Geometry: see drawing. Coordinates: mm, zero at the bounding-box minimum. A direction names the side the tool comes from. Give positions to 0.01 mm unless a question says otherwise; leave off trailing zeros. Write each loop counter-clockwise with the first axis right and the second up, starting at its lowest first coordinate (ties: lowest second). Pieces come first, ordered by that corner, then holes.
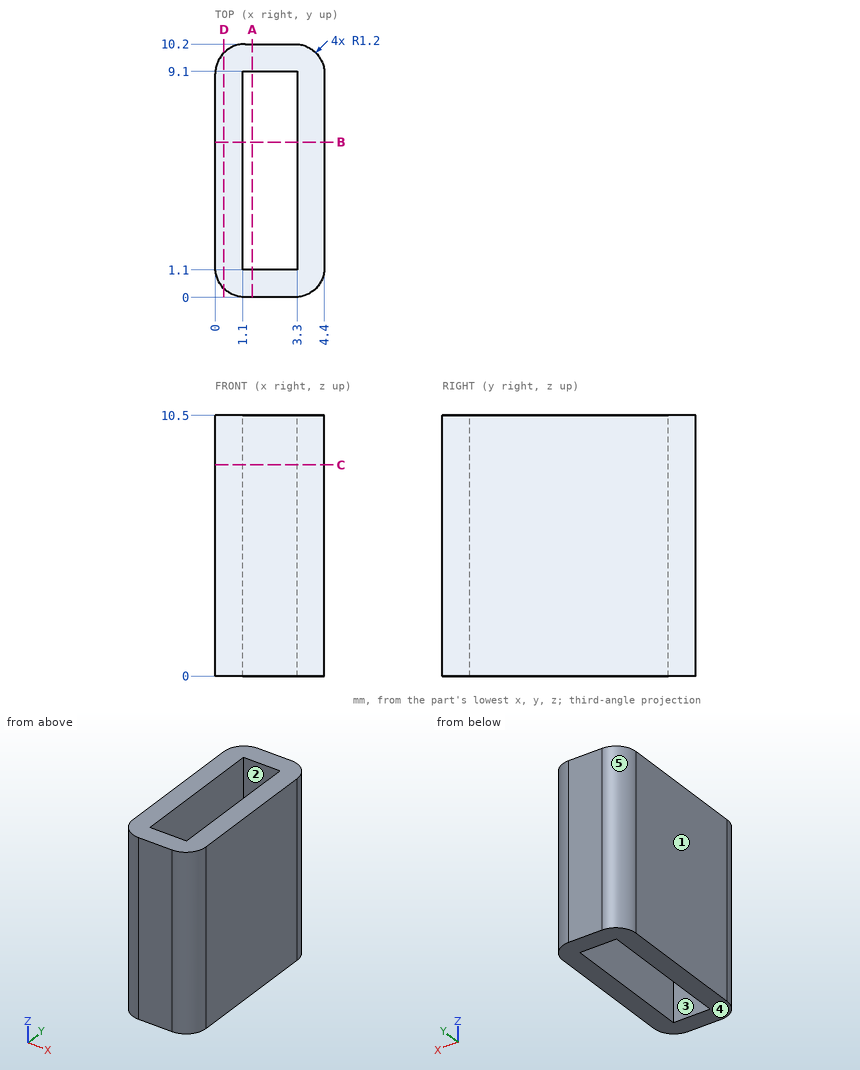
1. Section query A-A (x = 1.5). Return loops of the section in (y, z), plus the area to 3 significant figures.
2. Pull-direction query (X, two-part tool) for the marked faces 3, 4 and 5; classes: pulls with the +X half, pulls with the -X half, needs draft (parallel to the pull), parting line crosses it, or undercut.
3. Section query B-B (y = 6.25). Return loops of the section in (x, z).
4. Section query C-C (z = 8.5). Return loops of the section in (x, y), plus the area to 3 significant figures.
5. Line query: probe 1 along Y at (x, z) = (1.4, 2.75); probe 2 along X at (y, z) = (5.75, 3.5); probe 3 along Y at (x, z) = (0.5, 1.5). Output: solid intervals per line, ascending.
6. Access query for the marked faces 1 and 2. Directions: +Z, -Z, +X, -X, +Y, -Y. A direction counts if a zero-diameter tool reaches every point of the face in a straight line with its end or side. Return the directions, or none.
7. Section query D-D (x = 0.35). Return loops of the section in (y, z), plus the area to 3 significant figures.
8. Pin query (flat end, axial travel): P1, Ø4, axis at y = 6.5, z = 6.5, coming from the -X side. Return the tip coordinate at first contact, or that it passes through.
The answers:
1. outline: (0, 0) - (1.1, 0) - (1.1, 10.5) - (0, 10.5) - close; (9.1, 0) - (10.2, 0) - (10.2, 10.5) - (9.1, 10.5) - close
1. area: 23.1 mm2
2. face 3: undercut
2. face 4: needs draft
2. face 5: pulls with the -X half
3. outline: (0, 0) - (1.1, 0) - (1.1, 10.5) - (0, 10.5) - close; (3.3, 0) - (4.4, 0) - (4.4, 10.5) - (3.3, 10.5) - close
4. outline: (0, 1.2) arc R1.2 ccw to (1.2, 0) - (3.2, 0) arc R1.2 ccw to (4.4, 1.2) - (4.4, 9) arc R1.2 ccw to (3.2, 10.2) - (1.2, 10.2) arc R1.2 ccw to (0, 9) - close; hole (1.1, 1.1) - (3.3, 1.1) - (3.3, 9.1) - (1.1, 9.1) - close
4. area: 26.0 mm2
5. probe 1: y = 0 to 1.1, 9.1 to 10.2
5. probe 2: x = 0 to 1.1, 3.3 to 4.4
5. probe 3: y = 0.23 to 9.97
6. face 1: +Z, -Z, -X, +Y, -Y
6. face 2: +Z, -Z
7. outline: (0.35, 0) - (9.85, 0) - (9.85, 10.5) - (0.35, 10.5) - close
7. area: 99.7 mm2
8. P1: stops at x = 0
